from build123d import *

# Parameters (mm, degrees)
BOSS_EXTRUDE1_DEPTH                           = 1.5
BOSS_EXTRUDE1_DEPTH_BACK                      = 1.5
SKETCH1_W                                     = 110
SKETCH1_H                                     = 82.5
SKETCH1_R                                     = 2
SKETCH1_R_2                                   = 2.6
SKETCH1_W_2                                   = 50
SKETCH1_H_2                                   = 40
SKETCH2_W                                     = 30
SKETCH2_H                                     = 25
SKETCH2_R                                     = 4.3
SKETCH2_R_2                                   = 1.1
BOSS_EXTRUDE2_DEPTH                           = 3
FILLET1_R                                     = 3
ZIP_TIE_HOLES_AND_WEIGHT_REDUCTION_DEPTH      = 73.655436823
ZIP_TIE_HOLES_AND_WEIGHT_REDUCTION_DEPTH_BACK = 73.655436823
SKETCH3_R                                     = 2.5
SKETCH3_W                                     = 15
SKETCH3_H                                     = 25


with BuildPart() as part:
    # Sketch1 → Boss-Extrude1 (new, two sides: drawn at the far end of the back side and taken through both)
    with BuildSketch(Plane(origin=(0, 0, 0), x_dir=(1, 0, 0), z_dir=(0, 1, 0)).offset(-BOSS_EXTRUDE1_DEPTH_BACK)):
        Rectangle(SKETCH1_W, SKETCH1_H)
        with Locations(Location((45, 32.5, 0), (0, 0, 270))):
            Circle(SKETCH1_R, mode=Mode.SUBTRACT)
        with Locations(Location((45, -32.5, 0), (0, 0, 90))):
            Circle(SKETCH1_R, mode=Mode.SUBTRACT)
        with Locations(Location((-45, -32.5, 0), (0, 0, 270))):
            Circle(SKETCH1_R, mode=Mode.SUBTRACT)
        with Locations(Location((-45, 32.5, 0), (0, 0, 90))):
            Circle(SKETCH1_R, mode=Mode.SUBTRACT)
        with Locations(Location((-30, -25, 0), (0, 0, 270))):
            Circle(SKETCH1_R_2, mode=Mode.SUBTRACT)
        with Locations(Location((30, -25, 0), (0, 0, 90))):
            Circle(SKETCH1_R_2, mode=Mode.SUBTRACT)
        with Locations(Location((-30, 25, 0), (0, 0, 90))):
            Circle(SKETCH1_R_2, mode=Mode.SUBTRACT)
        with Locations(Location((30, 25, 0), (0, 0, 270))):
            Circle(SKETCH1_R_2, mode=Mode.SUBTRACT)
        Rectangle(SKETCH1_W_2, SKETCH1_H_2, mode=Mode.SUBTRACT)
    extrude(amount=BOSS_EXTRUDE1_DEPTH + BOSS_EXTRUDE1_DEPTH_BACK)

    # Sketch2 → Boss-Extrude2 (add)
    with BuildSketch(Plane(origin=(55, 0, 0), x_dir=(0, 0, -1), z_dir=(1, 0, 0))):
        with Locations((0, 11)):
            Rectangle(SKETCH2_W, SKETCH2_H)
        with Locations((0, 13.5)):
            Circle(SKETCH2_R, mode=Mode.SUBTRACT)
        with Locations((-4.75, 18.25)):
            Circle(SKETCH2_R_2, mode=Mode.SUBTRACT)
        with Locations(Location((4.75, 18.25, 0), (0, 0, 180))):
            Circle(SKETCH2_R_2, mode=Mode.SUBTRACT)
        with Locations((4.75, 8.75)):
            Circle(SKETCH2_R_2, mode=Mode.SUBTRACT)
        with Locations(Location((-4.75, 8.75, 0), (0, 0, 180))):
            Circle(SKETCH2_R_2, mode=Mode.SUBTRACT)
    extrude(amount=-BOSS_EXTRUDE2_DEPTH)

    # Fillet1
    fillet1_edges = [part.edges().sort_by_distance(p)[0] for p in [
        (52, 1.5, 0),
        (53.5, 1.5, -15),
        (53.5, 1.5, 15),
    ]]
    fillet(fillet1_edges, radius=FILLET1_R)

    # Sketch3 → Zip tie holes and weight reduction (cut, two sides: drawn at the far end of the back side and taken through both)
    with BuildSketch(Plane(origin=(0, 0, 0), x_dir=(1, 0, 0), z_dir=(0, 1, 0)).offset(-ZIP_TIE_HOLES_AND_WEIGHT_REDUCTION_DEPTH_BACK)):
        with Locations(Location((-10, -35.25, 0), (0, 0, 270))):
            Circle(SKETCH3_R)
        with Locations(Location((-10, -26, 0), (0, 0, 270))):
            Circle(SKETCH3_R)
        with Locations(Location((10, -26, 0), (0, 0, 90))):
            Circle(SKETCH3_R)
        with Locations(Location((10, -35.25, 0), (0, 0, 90))):
            Circle(SKETCH3_R)
        with Locations(Location((-10, 35.25, 0), (0, 0, 90))):
            Circle(SKETCH3_R)
        with Locations(Location((-10, 26, 0), (0, 0, 90))):
            Circle(SKETCH3_R)
        with Locations(Location((10, 26, 0), (0, 0, 270))):
            Circle(SKETCH3_R)
        with Locations(Location((10, 35.25, 0), (0, 0, 270))):
            Circle(SKETCH3_R)
        with Locations((40, 0)):
            Rectangle(SKETCH3_W, SKETCH3_H)
        with Locations((-40, 0)):
            Rectangle(SKETCH3_W, SKETCH3_H)
    extrude(amount=ZIP_TIE_HOLES_AND_WEIGHT_REDUCTION_DEPTH + ZIP_TIE_HOLES_AND_WEIGHT_REDUCTION_DEPTH_BACK, mode=Mode.SUBTRACT)


solid = part.part
Could you check a few things on this model? Use its own coordinates, in mm. A direction names the side the tool comes from. Give positions to 0.01 mm unless a question says otherwise; leave off trailing zeros. Order: outer loops, then holes, each group sorted by start corner. A loop starts at its lowest first (then second) coordinate and runs counter-clockwise, first axis right, second up.
1. Suppose I cut it at A-A (y = 13.5). List the corners of the cut face in (x, z) for me, plus the area to 3 significant figures.
2. For faces 4 (the cylindrical face through (53.521, 17.176, 4.988)), 5 (the flat face through (25, 0, 0)), 6 (the flat face through (54, 14, 15)), which set-ups out of +Z, -Z, +X, -X, +Y, -Y let a thin tool reach every point of the face, with its end or its side?
3. We'd pull the mould along Z, two halves only. Please class faces 1 (the flat face through (-40, 0, 12.5)), 2 (the cylindrical face through (52.62, 2.02, 16.31)), 3 (the flat face through (52, 16, 4)): pulls with the +Z half, pulls with the -Z half, needs draft (parallel to the pull), parting line crosses it, or undercut.
4. Suppose I cut it at D-D (x = 39.5). List the corners of the cut face in (y, z) for me.
5. Will these pins go through, and if not, where does the flat tip stop? P1, Ø3.5, axis at x = 53.5, y = 16, coming from the -Z side; P2, Ø6, axis at x = -10, z = 26, coming from the +Y side; P3, Ø3, axis at y = 17, z = 4, coming from the -X side; P4, Ø1.5, axis at y = 10.5, z = 0, coming from the +X side.
6. I need wall thicknesses on L1, parallel to X at y = -0.8, z = 32.5; L2, parallel to X at y = 0.45, z = 26; L3, parallel to Z at x = 13.5, y = 0. Which ranges of each line are inside material? Lowest first, please.
7. Suppose I cut it at B-B (x = -45). List the corners of the cut face in (y, z) for me, plus the area to 4 significant figures.
8. Suppose I cut it at C-C (z = 8). List the corners of the cut face in (x, y) for me, plus the area to 3 significant figures.
Solved:
1. outline: (52, -15) - (55, -15) - (55, -4.3) - (52, -4.3) - close; (52, 4.3) - (55, 4.3) - (55, 15) - (52, 15) - close
1. area: 64.2 mm2
2. face 4: +X, -X
2. face 5: +Y, -Y
2. face 6: +Z, +X, -X, +Y
3. face 1: undercut
3. face 2: pulls with the +Z half
3. face 3: needs draft
4. outline: (-1.5, -41.25) - (1.5, -41.25) - (1.5, -12.5) - (-1.5, -12.5) - close; (-1.5, 12.5) - (1.5, 12.5) - (1.5, 41.25) - (-1.5, 41.25) - close
5. P1: stops at z = -15
5. P2: stops at y = 1.5
5. P3: stops at x = 52
5. P4: passes through
6. L1: x = -55 to -47, -43 to 43, 47 to 55
6. L2: x = -55 to -32.4, -27.6 to -12.5, -7.5 to 7.5, 12.5 to 27.6, 32.4 to 55
6. L3: z = -41.25 to -20, 20 to 41.25
7. outline: (-1.5, -41.25) - (1.5, -41.25) - (1.5, -34.5) - (-1.5, -34.5) - close; (-1.5, -30.5) - (1.5, -30.5) - (1.5, -12.5) - (-1.5, -12.5) - close; (-1.5, 12.5) - (1.5, 12.5) - (1.5, 30.5) - (-1.5, 30.5) - close; (-1.5, 34.5) - (1.5, 34.5) - (1.5, 41.25) - (-1.5, 41.25) - close
7. area: 148.5 mm2
8. outline: (-55, -1.5) - (-47.5, -1.5) - (-47.5, 1.5) - (-55, 1.5) - close; (-32.5, -1.5) - (-25, -1.5) - (-25, 1.5) - (-32.5, 1.5) - close; (25, -1.5) - (32.5, -1.5) - (32.5, 1.5) - (25, 1.5) - close; (47.5, -1.5) - (55, -1.5) - (55, 23.5) - (52, 23.5) - (52, 4.5) arc R3 cw to (49, 1.5) - (47.5, 1.5) - close
8. area: 158 mm2
